Build history of the part. All positions in model axes, mm. A direction names the side the tool comes from. Give positions to 0.01 mm unless a question says otherwise; leave off trailing zeros. Loops run counter-clockwise (first coordinate to the right, second up) from the corner with the lowest first, then second, coordinate; pieces in that order, holes last. Notation, with made-up numbers: (11.5, -29) - (29.5, -29) arc R34 ccw to (29.5, 8) - close; hole circle Ø4 at (0, 82). An arc over 180 degrees is marked (long way). Return JSON: item names as keys, results as strings. Group by question number.
1) Slice it at C-C (z = -2.5). List the corners of the cut face in (x, y), and give its area (3 significant figures).
2) Slice it at D-D (y = 7.25). List the corners of the cut face in (x, z), and give its area (3 significant figures).
3) Slice it at A-A (x = -7.75). List the corners of the cut face in (y, z), and give its area (3 significant figures).
4) Drill centre lines: probe 1 along Z at (x, y) = (-1, 8.25); probe 2 along X at (y, z) = (-1.75, -1.5); probe 3 along X at (y, z) = (1, 22). Where is each one in solid material? Low to high. Write a range as from..to.
5) 3-axis set-ups, long thin cutter, end or side, ignore diameter. For faces 1 (the face through (15, 0, 10)), 2 (the face through (-3.754, 0.176, -2.465)), 3 (the face through (-3.754, 0.176, 22.465)): which of +Z, -Z, +X, -X, +Y, -Y reach the whole face in a straight line?
6) Slice it at B-B (y = 0). List the corners of the cut face in (x, z), and give its area (3 significant figures).
7) Drop a flat-ended pin along its axis: pin 1 (9 mm diameter, centred on x = 6.5, y = 2, fed in from -Z). Give the stop position or say it passes through.
```python
from build123d import *

# Parameters (mm, degrees)
ESQUISSE1_W        = 30
ESQUISSE1_H        = 18
BOSS_EXTRU_1_DEPTH = 20
ESQUISSE2_R        = 4
BOSS_EXTRU_2_DEPTH = 5


with BuildPart() as part:
    # Esquisse1 → Boss.-Extru.1 (new body)
    with BuildSketch(Plane.XY):
        Rectangle(ESQUISSE1_W, ESQUISSE1_H)
    extrude(amount=BOSS_EXTRU_1_DEPTH)

    # Esquisse2 → Boss.-Extru.2 (add)
    with BuildSketch(Plane(origin=(0, 0, 0), x_dir=(-1, 0, 0), z_dir=(0, 0, -1))):
        with Locations((7.75, 0)):
            Circle(ESQUISSE2_R)
    boss_extru_2 = extrude(amount=BOSS_EXTRU_2_DEPTH)

    # Symétrie1: Boss.-Extru.2 across plane
    add(boss_extru_2.mirror(Plane.XY.offset(10)))


solid = part.part
```
Results:
{
 "1": {"outline": "circle Ø8 at (-7.75, 0)", "area": "50.3 mm2"},
 "2": {"outline": "(-15, 0) - (15, 0) - (15, 20) - (-15, 20) - close", "area": "600 mm2"},
 "3": {"outline": "(-9, 0) - (-4, 0) - (-4, -5) - (4, -5) - (4, 0) - (9, 0) - (9, 20) - (4, 20) - (4, 25) - (-4, 25) - (-4, 20) - (-9, 20) - close", "area": "440 mm2"},
 "4": {"probe 1": "0..20", "probe 2": "-11.35..-4.15", "probe 3": "-11.62..-3.88"},
 "5": {"face 1": "+Z, -Z, +X, +Y, -Y", "face 2": "-Z", "face 3": "+Z"},
 "6": {"outline": "(-15, 0) - (-11.75, 0) - (-11.75, -5) - (-3.75, -5) - (-3.75, 0) - (15, 0) - (15, 20) - (-3.75, 20) - (-3.75, 25) - (-11.75, 25) - (-11.75, 20) - (-15, 20) - close", "area": "680 mm2"},
 "7": {"pin 1": "z = 0"}
}
